from build123d import *

# Parameters (mm, degrees)
SKETCH2_R           = 30
BOSS_EXTRUDE1_DEPTH = 125
CUT_EXTRUDE1_START  = -50
CUT_EXTRUDE1_DEPTH  = 50
CUT_EXTRUDE2_START  = -50
CUT_EXTRUDE2_DEPTH  = 50


with BuildPart() as part:
    # Sketch2 → Boss-Extrude1 (new, symmetric)
    with BuildSketch(Plane(origin=(0, 0, 0), x_dir=(1, 0, 0), z_dir=(0, 1, 0))):
        with Locations(Location((0, 0, 0), (0, 0, 270))):
            Circle(SKETCH2_R)
    extrude(amount=BOSS_EXTRUDE1_DEPTH, both=True)

    # Sketch3 → Cut-Extrude1 (cut)
    with BuildSketch(Plane.XZ.offset(125).offset(CUT_EXTRUDE1_START)):
        with BuildLine():
            ThreePointArc((-8.095335695, 28.887117197), (0, 30), (8.095335695, 28.887117197))
            Line((8.095335695, 28.887117197), (8.095335695, 34.42))
            Line((8.095335695, 34.42), (-8.095335695, 34.42))
            Line((-8.095335695, 34.42), (-8.095335695, 28.887117197))
        make_face()
        with BuildLine():
            Line((-8.095335695, 27.42), (8.095335695, 27.42))
            Line((8.095335695, 27.42), (8.095335695, 28.887117197))
            ThreePointArc((8.095335695, 28.887117197), (0, 30), (-8.095335695, 28.887117197))
            Line((-8.095335695, 28.887117197), (-8.095335695, 27.42))
        make_face()
    extrude(amount=CUT_EXTRUDE1_DEPTH, mode=Mode.SUBTRACT)

    # Sketch4 → Cut-Extrude2 (cut)
    with BuildSketch(Plane(origin=(0, -15, 0), x_dir=(-1, 0, 0), z_dir=(0, -1, 0)).offset(CUT_EXTRUDE2_START)):
        with BuildLine():
            Line((8.095335695, -28.887117197), (8.095335695, -27.42))
            Line((8.095335695, -27.42), (-8.095335695, -27.42))
            Line((-8.095335695, -27.42), (-8.095335695, -28.887117197))
            ThreePointArc((-8.095335695, -28.887117197), (0, -30), (8.095335695, -28.887117197))
        make_face()
    extrude(amount=CUT_EXTRUDE2_DEPTH, mode=Mode.SUBTRACT)


solid = part.part
Build history of the part. All positions in model axes, mm. A direction names the side the tool comes from. Give positions to 0.01 mm unless a question says otherwise; leave off trailing zeros. Order: outer loops, then holes, each group sorted by start corner. A loop starts at its lowest first (then second) coordinate and runs counter-clockwise, first axis right, second up. Notation, with made-up numbers: M 57.25,20.25 L 79.25,20.25 A18 ccw 79.25,42.25 Z; hole C 84.5,65.5 d5. An arc over 180 degrees is marked long. Put each result on its own line as item: value.
Item 1: Slice it at B-B, the plane y = 96. Write the cut outline in (x, z).
From the geometry:
outline: C 0,0 d60
Item 2: Slice it at A-A, the plane x = 0. Write the cut outline in (y, z).
From the geometry:
outline: M -125,-30 L 125,-30 L 125,30 L 35,30 L 35,27.42 L -15,27.42 L -15,30 L -75,30 L -75,27.42 L -125,27.42 Z
Item 3: Slice it at C-C, the plane z = -12. Write the cut outline in (x, y).
From the geometry:
outline: M -27.5,-125 L 27.5,-125 L 27.5,125 L -27.5,125 Z
Item 4: Slice it at D-D, the plane x = 20.5. Write the cut outline in (y, z), plus the area to 3 significant figures.
From the geometry:
outline: M -125,-21.9 L 125,-21.9 L 125,21.9 L -125,21.9 Z
area: 11,000 mm2
Item 5: Two-plate mould, pull along X, no slides. Class faces 1 (the cylindrical face through (-11.49, 1.75, 27.712)), 2 (the flat face through (0, 125, 0)), 3 (the flat face through (0, 10, 27.42)): +X half, -X half, draft (parallel to the pull), parting line (faces both ways), or undercut.
From the geometry:
face 1: parting line
face 2: draft
face 3: undercut
Item 6: 3-axis set-ups, long thin cutter, end or side, ignore diameter. For faces 4 (the flat face through (0, -100, 27.42)), 5 (the flat face through (0, -125, -1)): which of +Z, -Z, +X, -X, +Y, -Y reach the whole face in a straight line?
From the geometry:
face 4: +Z, -Y
face 5: +Z, -Z, +X, -X, -Y
Item 7: Probe line 1 (Z direction, x = -3, y = -9); line 2 (X direction, y = 33.5, z = -17.5); line 3 (Z direction, x = -21.5, y = 0). List the from-to ranges inside material, lowest first. Write a range as [from, to].
From the geometry:
line 1: z = [-29.85, 27.42]
line 2: x = [-24.37, 24.37]
line 3: z = [-20.92, 20.92]
Item 8: Flat gauge pins, fed straight in: pin 1 Ø1.2 at (y, z) = (-98.5, 28) entering from +X; pin 2 Ø3 at (x, y) = (-15.5, -62) entering from -Z; pin 3 Ø3 at (y, z) = (35, 7) entering from +X; pin 4 Ø12 at (x, y) = (-3, -73) entering from +Z. Where does each tip first touch, or does it go through?
From the geometry:
pin 1: stops at x = 12.22
pin 2: stops at z = -26.53
pin 3: stops at x = 29.49
pin 4: stops at z = 30
